The drawing under review shows one solid part. Ordinate dimensions are in mm from its lowest x, y, z. Give positions to 0.01 mm unless a question says otherwise; leave off trailing zeros. Write each loop counter-clockwise with the first axis right and the second up, starting at its lowest first coordinate (ties: lowest second). Pieces come first, ordered by that corner, then holes.
Q1. For line 1 (Y direction, x = 67.5, z = 1.05) (3 decimals); line 2 (X direction, y = 153.75, z = 0.7) (3 decimals); line 3 (Y direction, x = 10, z = 1.95) (3 decimals), list the stretches that pass through material, from the lowest coordinate up.
Q2. We need section A-A (z = 1.75). Give the number of separate pieces and of enclosed holes in the cut face, then the cut area to 3 significant figures.
Q3. We need section B-B (y = 140.5). Write out the cut boundary in (x, z) (3 decimals).
Q4. Insertion check: P1, Ø1, axis at x = 88.5, z = 1.5, coming from the -Y side; P2, Ø1, axis at x = 75, z = 1.5, coming from the +Y side (3 decimals); P3, Ø1.6, axis at x = 2, z = 1, coming from the +Y side. Each pin has a flat end and moves straight along its axis. Give the tip position at first contact, or say it passes through.
Q5. We need section C-C (x = 15.5). Write out the cut boundary in (y, z) (3 decimals), then the cut area to 3 significant figures.
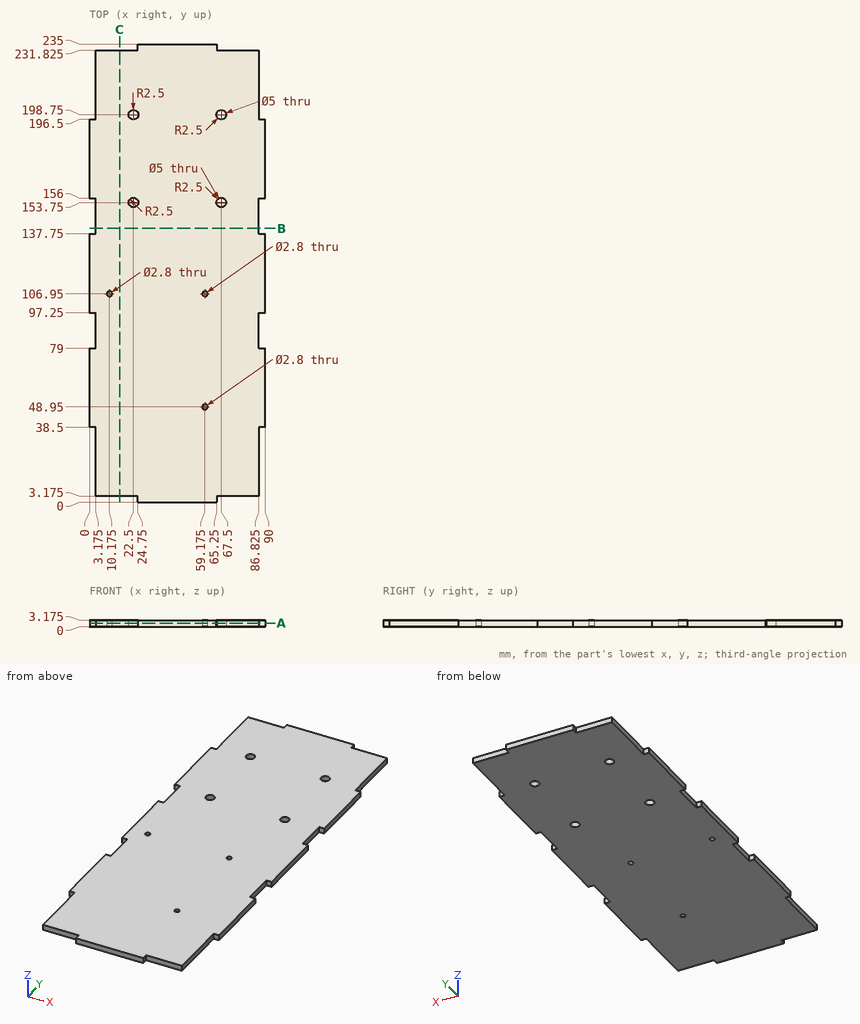
Computed:
1. line 1: y = 3.175 to 151.25, 156.25 to 196.25, 201.25 to 231.825
1. line 2: x = 3.175 to 20, 25 to 65, 70 to 86.825
1. line 3: y = 3.175 to 105.561, 108.339 to 231.825
2. separate pieces: 1
2. enclosed holes: 7
2. area: 20,100 mm2
3. outline: (3.175, 0) - (86.825, 0) - (86.825, 3.175) - (3.175, 3.175) - close
4. P1: stops at y = 38.5
4. P2: stops at y = 231.825
4. P3: stops at y = 196.5
5. outline: (3.175, 0) - (231.825, 0) - (231.825, 3.175) - (3.175, 3.175) - close
5. area: 726 mm2
